```python
from build123d import *

# Parameters (mm, degrees)
F0_R     = 11
F0_R_2   = 1.75
F0_R_3   = 3.5
F1_DEPTH = 3.5
F2_DEPTH = 2.6
F3_W     = 22
F3_H     = 22
F4_DEPTH = 25


with BuildPart() as f1:
    # F0 (on Top) → F1 (new body, symmetric)
    with BuildSketch(Plane.XY):
        Circle(F0_R)
        with Locations((0, -8)):
            Circle(F0_R_2, mode=Mode.SUBTRACT)
        Polygon((-2.847942, -5.351563), (-6.05856, -0.209391), (-3.210618, 5.142172), (2.847942, 5.351563), (6.05856, 0.209391), (3.210618, -5.142172), align=None, mode=Mode.SUBTRACT)
        with Locations((0, 8)):
            Circle(F0_R_2, mode=Mode.SUBTRACT)
        Polygon((-3.210618, 5.142172), (-6.05856, -0.209391), (-2.847942, -5.351563), (3.210618, -5.142172), (6.05856, 0.209391), (2.847942, 5.351563), align=None)
        Circle(F0_R_3, mode=Mode.SUBTRACT)
    extrude(amount=F1_DEPTH, both=True)

    # F0 (on Top) → F2 (cut, symmetric)
    with BuildSketch(Plane.XY):
        Polygon((-3.210618, 5.142172), (-6.05856, -0.209391), (-2.847942, -5.351563), (3.210618, -5.142172), (6.05856, 0.209391), (2.847942, 5.351563), align=None)
        Circle(F0_R_3, mode=Mode.SUBTRACT)
    extrude(amount=F2_DEPTH, both=True, mode=Mode.SUBTRACT)

    # F3 (on Top) → F4 (cut)
    with BuildSketch(Plane.XY):
        Rectangle(F3_W, F3_H)
    extrude(amount=F4_DEPTH, mode=Mode.SUBTRACT)


solid = f1.part
```
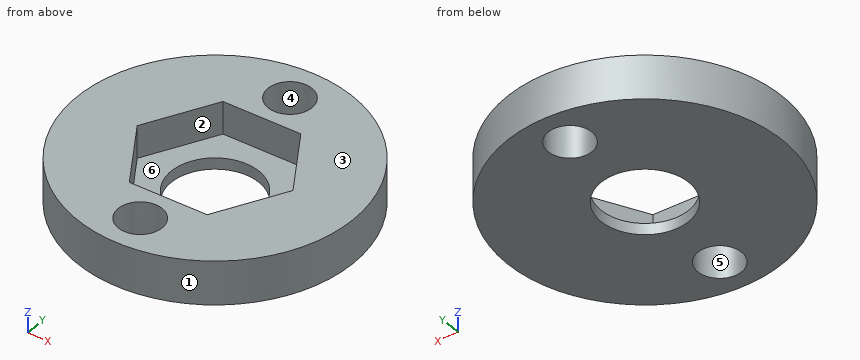
Here's how the part is built. I have some questions about the finished solid (model axes, mm). Face numbers are marked on the shaded views. A direction names the side the tool comes from. Round coordinates to 2 decimals unless told otherwise and drop trailing zeros. Write each loop counter-clockwise with the first axis right and the second up, starting at its lowest first coordinate (ties: lowest second). Pieces come first, ordered by that corner, then holes.
Q1. If we section it at A-A on z = -2.3: Write out the boundary of the cut face in (x, y), plus the area to 3 significant figures.
Q2. If we section it at D-D on y = -1: Write out the boundary of the cut face in (x, z), plus the area to 3 significant figures.
Q3. Will these pins go through, and if not, where does the flat tip stop? P1, Ø3, axis at x = 0, y = 8, coming from the +Z side; P2, Ø1.5, axis at y = 1, z = -1, coming from the -X side; P3, Ø1.5, axis at x = 4, z = -2.5, coming from the +Y side; P4, Ø5.5, axis at x = -2.5, y = 0.5, coming from the +Z side.
Q4. If we section it at C-C on x = 0: Write out the boundary of the cut face in (y, z), plus the area to 3 significant figures.
Q5. Please list where these lines run through material, in increasing order: probe 1 along Y at (x, z) = (0, -2.5); probe 2 along Y at (x, z) = (0, -2.75); probe 3 along Z at (x, y) = (4.5, 1.5).
Q6. If we mould it in two halves opening along Y, with no side actions, what happens to the marked faces 1, 2, 3 and 4? For each: +Y half, -Y half, draft (parallel to the pull), parting line (faces both ways), or undercut.
Q7. Which directions (+Z, -Z, +X, -X, +Y, -Y) give clear straight access to the entire face, cutting with the end or side of a thin tool? Please do the marked faces 5 and 6.
Q8. If we section it at B-B on y = 8: Write out the boundary of the cut face in (x, z).
Answer below:
1. outline: circle Ø22 at (0, 0); hole (-6.06, -0.21) - (-2.85, -5.35) - (3.21, -5.14) - (6.06, 0.21) - (2.85, 5.35) - (-3.21, 5.14) - close; hole circle Ø3.5 at (0, -8); hole circle Ø3.5 at (0, 8)
1. area: 265 mm2
2. outline: (-10.95, -3.5) - (-3.35, -3.5) - (-3.35, -2.6) - (-5.56, -2.6) - (-5.56, 0) - (-10.95, 0) - close; (3.35, -3.5) - (10.95, -3.5) - (10.95, 0) - (5.41, 0) - (5.41, -2.6) - (3.35, -2.6) - close
2. area: 42.1 mm2
3. P1: passes through
3. P2: stops at x = -11
3. P3: stops at y = 10.51
3. P4: stops at z = -2.6
4. outline: (-11, -3.5) - (-9.75, -3.5) - (-9.75, 0) - (-11, 0) - close; (-6.25, -3.5) - (-3.5, -3.5) - (-3.5, -2.6) - (-5.25, -2.6) - (-5.25, 0) - (-6.25, 0) - close; (3.5, -3.5) - (6.25, -3.5) - (6.25, 0) - (5.25, 0) - (5.25, -2.6) - (3.5, -2.6) - close; (9.75, -3.5) - (11, -3.5) - (11, 0) - (9.75, 0) - close
4. area: 18.9 mm2
5. probe 1: y = -11 to -9.75, -6.25 to -5.25, 5.25 to 6.25, 9.75 to 11
5. probe 2: y = -11 to -9.75, -6.25 to -3.5, 3.5 to 6.25, 9.75 to 11
5. probe 3: z = -3.5 to -2.6
6. face 1: parting line
6. face 2: undercut
6. face 3: draft
6. face 4: undercut
7. face 5: +Z, -Z
7. face 6: +Z
8. outline: (-7.55, -3.5) - (-1.75, -3.5) - (-1.75, 0) - (-7.55, 0) - close; (1.75, -3.5) - (7.55, -3.5) - (7.55, 0) - (1.75, 0) - close
